Source: CAD feature listing. Evaluate the final solid. Frame: model axes, mm. Give positions to 0.01 mm unless a question says otherwise; leave off trailing zeros. Order: outer loops, then holes, each group sorted by start corner. A loop starts at its lowest first (then second) coordinate and runs counter-clockwise, first axis right, second up. Notation, with made-up numbers: (-5.75, 62) -> (40.25, 62) arc R23 cw to (40.25, 86) -> close; hole circle Ø4 at (31, 74). An arc over 180 degrees is marked (long way). Answer in a Markdown table with one row per item.
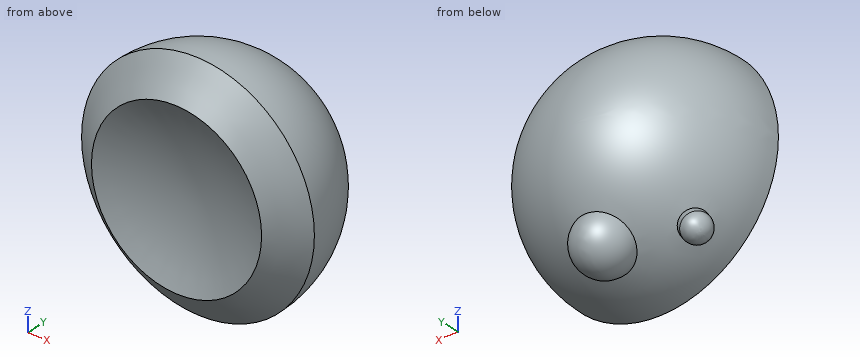
```python
from build123d import *


with BuildPart() as part:
    # Sketch 1 → Revolve 1 (revolve)
    with BuildSketch(Plane.XY):
        with BuildLine():
            Line((-75, 129.232052778), (-54.801890605, 112.34657443))
            ThreePointArc((-54.801890605, 112.34657443), (-28.12186157, 121.795570124), (0, 125))
            Line((0, 125), (0, 204.232052778))
            ThreePointArc((0, 204.232052778), (-53.033008589, 182.265061367), (-75, 129.232052778))
        make_face()
    revolve(axis=Axis((0, 213.081349398, 0), (0, -1, 0)))

    # Sketch 6 → Revolve 2 (revolve)
    with BuildSketch(Plane(origin=(0, 0, 0), x_dir=(0, 0, -1), z_dir=(1, 0, 0))):
        with BuildLine():
            Line((36.229745399, 174.39946224), (73.229745399, 174.39946224))
            ThreePointArc((73.229745399, 174.39946224), (54.729745399, 192.89946224), (36.229745399, 174.39946224))
        make_face()
    revolve(axis=Axis((0, 174.39946224, 0), (0, 0, -1)))

    # Sketch 9 → Revolve 4 (revolve)
    with BuildSketch(Plane(origin=(0, 0, 0), x_dir=(0, 1, 0), z_dir=(-0.766518382, 0, 0.642222368))):
        with BuildLine():
            Line((156.556180661, 65.879169876), (163.258797924, 82.039351206))
            ThreePointArc((163.258797924, 82.039351206), (156.56373545, 82.042480502), (151.827398627, 77.310569172))
            Line((151.827398627, 77.310569172), (148.476089996, 69.230478507))
            Line((148.476089996, 69.230478507), (156.556180661, 65.879169876))
        make_face()
    revolve(axis=Axis((0, 129.232052778, 0), (-0.593221163, 0.383115215, -0.708033462)))

    # Sketch 15 → Revolve 5 (revolve)
    with BuildSketch(Plane.XY):
        with BuildLine():
            Line((0, 125), (0, -125))
            ThreePointArc((0, -125), (125, 0), (0, 125))
        make_face()
    revolve(axis=Axis((0, 143.905509185, 0), (0, -1, 0)))

    # Sketch 15_3 → Cut-Revolve 5 (revolve, cut)
    with BuildSketch(Plane.XY):
        with BuildLine():
            Line((0, 125), (0, -125))
            ThreePointArc((0, -125), (125, 0), (0, 125))
        make_face()
    revolve(axis=Axis((0, 143.905509185, 0), (0, -1, 0)), mode=Mode.SUBTRACT)


solid = part.part
```
(1) Section query B-B (x = 0). Return the cut outline in (y, z).
A:
| item | result |
|---|---|
| outline | (112.35, -54.8) -> (129.23, -75) arc R75 ccw to (161.3, -67.8) arc R18.5 ccw to (189.71, -44.35) arc R75 ccw to (129.23, 75) -> (112.35, 54.8) arc R125 cw to start |
(2) Section query C-C (y = 142). Return the cut outline in (x, z).
A:
| item | result |
|---|---|
| outline | circle Ø147.81 at (0, 0) |
(3) Ray query, probe 1 along Z at (x, y) = (-34.5, 167); probe 2 along Z at (x, y) = (-31, 128); probe 3 along Y at (x, z) = (-61, -0.5). Return the intervals inside material, ascending.
A:
| item | result |
|---|---|
| probe 1 | z = -54.85 to 54.85 |
| probe 2 | z = -66.67 to 66.67 |
| probe 3 | y = 117.53 to 172.86 |
(4) Section query A-A (z = 0). Return the cut outline in (x, y), plus the area to 3 significant figures.
A:
| item | result |
|---|---|
| outline | (-75, 129.23) -> (-54.8, 112.35) arc R125 cw to (54.8, 112.35) -> (75, 129.23) arc R75 ccw to start |
| area | 10,100 mm^2 |
(5) First-contact query: pin 1 Ø8 at (y, z) = (147.5, 57.5) entering from -X; pin 2 Ø3 at (x, z) = (13.5, 55.5) entering from +Y; pin 3 Ø10 at (x, z) = (42.5, 59.5) entering from +Y. Flat tips, straight axial feed; report the tip coordinate or a pass-through.
A:
| item | result |
|---|---|
| pin 1 | stops at x = -49.51 |
| pin 2 | stops at y = 179.55 |
| pin 3 | stops at y = 160.61 |
(6) Section query D-D (y = 196). Return the cut outline in (x, z).
A:
| item | result |
|---|---|
| outline | circle Ø68.32 at (0, 0) |
